Build history of the part. All positions in model axes, mm. Round coordinates to 2 decimals unless told otherwise and drop trailing zeros. Write each loop counter-clockwise with the first axis right and the second up, starting at its lowest first coordinate (ties: lowest second). Pieces come first, ordered by that corner, then holes. Notation, with made-up numbers: (-10.75, 50) -> (32.25, 50) arc R17 cw to (32.25, 83) -> close; hole circle Ø5 at (52, 88). An arc over 180 degrees is marked (long way). Answer in a Markdown table with one row per item.
```python
from build123d import *

# Parameters (mm, degrees)
SKETCH1_R                            = 3
SKETCH1_R_2                          = 2.55
BOSS_EXTRUDE1_DEPTH                  = 18.47
CUT_EXTRUDE1_DEPTH                   = 19.951013166
CUT_EXTRUDE1_DEPTH_BACK              = 19.951013166
SKETCH2_W                            = 0.254
SKETCH2_H                            = 13
F_0_6_0_6_DIAMETER_HOLE1_D           = 0.6
F_0_6_0_6_DIAMETER_HOLE1_ON_FACE_2_D = 0.6
F_0_6_0_6_DIAMETER_HOLE1_ON_FACE_3_D = 0.6
F_0_6_0_6_DIAMETER_HOLE1_ON_FACE_4_D = 0.6


with BuildPart() as part:
    # Sketch1 → Boss-Extrude1 (new body)
    with BuildSketch(Plane(origin=(0, 0, 0), x_dir=(1, 0, 0), z_dir=(0, 1, 0))):
        with Locations(Location((0, 0, 0), (0, 0, 270))):
            Circle(SKETCH1_R)
        with Locations(Location((0, 0, 0), (0, 0, 270))):
            Circle(SKETCH1_R_2, mode=Mode.SUBTRACT)
    extrude(amount=BOSS_EXTRUDE1_DEPTH)

    # Sketch2 → Cut-Extrude1 (cut, two sides: drawn at the far end of the back side and taken through both)
    with BuildSketch(Plane.XY.offset(-CUT_EXTRUDE1_DEPTH_BACK)):
        with Locations((0, 11.97)):
            Rectangle(SKETCH2_W, SKETCH2_H)
    extrude(amount=CUT_EXTRUDE1_DEPTH + CUT_EXTRUDE1_DEPTH_BACK, mode=Mode.SUBTRACT)

    # Ø0.6 (0.6) Diameter Hole1 (through all)
    with Locations(Plane(origin=(2.121320344, 17.97, 2.121320344), x_dir=(0.707106781187, 0, -0.707106781187), z_dir=(0.707106781187, 0, 0.707106781187))):
        with Locations((0, 0)):
            Hole(F_0_6_0_6_DIAMETER_HOLE1_D / 2)

    # Ø0.6 (0.6) Diameter Hole1 on face 2 (through all)
    with Locations(Plane(origin=(2.121320344, 17.97, -2.121320344), x_dir=(-0.707106781187, 0, -0.707106781187), z_dir=(0.707106781187, 0, -0.707106781187))):
        with Locations((0, 0)):
            Hole(F_0_6_0_6_DIAMETER_HOLE1_ON_FACE_2_D / 2)

    # Ø0.6 (0.6) Diameter Hole1 on face 3 (through all)
    with Locations(Plane(origin=(-2.121320344, 17.97, 2.121320344), x_dir=(0.707106781187, 0, 0.707106781187), z_dir=(-0.707106781187, 0, 0.707106781187))):
        with Locations((0, 0)):
            Hole(F_0_6_0_6_DIAMETER_HOLE1_ON_FACE_3_D / 2)

    # Ø0.6 (0.6) Diameter Hole1 on face 4 (through all)
    with Locations(Plane(origin=(-2.121320344, 17.97, -2.121320344), x_dir=(-0.707106781187, 0, 0.707106781187), z_dir=(-0.707106781187, 0, -0.707106781187))):
        with Locations((0, 0)):
            Hole(F_0_6_0_6_DIAMETER_HOLE1_ON_FACE_4_D / 2)


solid = part.part
```
Q1. Saw through at A-A on y = 16.25. Write the cut outline in (x, z).
A:
| item | result |
|---|---|
| outline | (-0.13, -3) -> (-0.13, -2.55) arc R2.55 cw to (-0.13, 2.55) -> (-0.13, 3) arc R3 ccw to start; (0.13, -3) arc R3 ccw to (0.13, 3) -> (0.13, 2.55) arc R2.55 cw to (0.13, -2.55) -> close |
Q2. Drop flat-ended pins along their axis: P1, Ø3, axis at x = 2.5, y = 16, coming from the +Z side; P2, Ø0.5, axis at y = 10, z = 2.5, coming from the +X side; P3, Ø2, axis at y = 12, z = -2.5, coming from the -X side. Give the stop position or say it passes through.
A:
| item | result |
|---|---|
| P1 | z = 2.83 |
| P2 | x = 1.98 |
| P3 | x = -2.6 |
Q3. Two-plate mould, pull along Z, no slides. Class faces 1 (the flat face through (-2.7, 18.47, -0.2)), 2 (the cylindrical face through (0.9, 9.11, 2.86)), 3 (the cylindrical face through (0.77, 9.11, 2.43)): released by +Z, released by -Z, zero draft, split by the parting line, or undercut.
A:
| item | result |
|---|---|
| face 1 | zero draft |
| face 2 | split by the parting line |
| face 3 | undercut |
Q4. Saw through at C-C on y = 1.5. Write the cut outline in (x, z), plus the area to 3 significant figures.
A:
| item | result |
|---|---|
| outline | circle Ø6 at (0, 0); hole circle Ø5.1 at (0, 0) |
| area | 7.85 mm² |
Q5. Saw through at B-B on z = 0. Write the cut outline in (x, y), plus the area to 3 significant figures.
A:
| item | result |
|---|---|
| outline | (-3, 0) -> (-2.55, 0) -> (-2.55, 18.47) -> (-3, 18.47) -> close; (2.55, 0) -> (3, 0) -> (3, 18.47) -> (2.55, 18.47) -> close |
| area | 16.6 mm² |
Q6. Wall check: line 1 (X direction, y = 12, z = 0); line 2 (X direction, y = 17.25, z = 1.5). Give the ranges that are in metal, low to high. Write a range as [from, to].
A:
| item | result |
|---|---|
| line 1 | [-3, -2.55], [2.55, 3] |
| line 2 | [-2.6, -2.06], [2.06, 2.6] |
